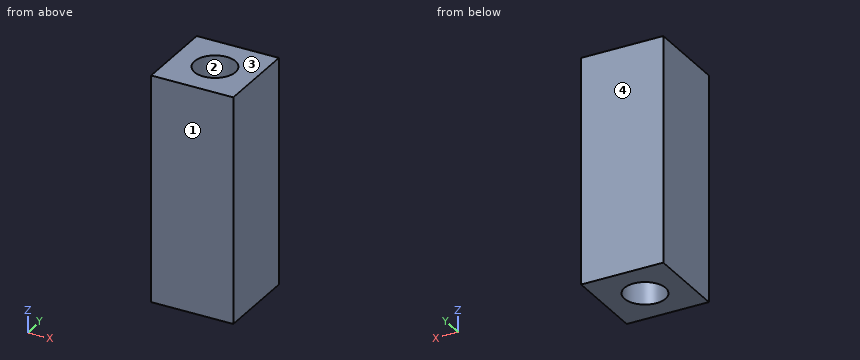
```python
from build123d import *

# Parameters (mm, degrees)
F1_DEPTH = 279.4


with BuildPart() as f1:
    # F0 (on Top) → F1 (new body)
    with BuildSketch(Plane.XY):
        with BuildLine():
            ThreePointArc((-25.4, 0), (0, 25.4), (25.4, 0))
            Line((25.4, 0), (50.8, 0))
            Line((50.8, 0), (50.8, 50.8))
            Line((50.8, 50.8), (-50.8, 50.8))
            Line((-50.8, 50.8), (-50.8, 0))
            Line((-50.8, 0), (-25.4, 0))
        make_face()
        with BuildLine():
            Line((50.8, 0), (25.4, 0))
            ThreePointArc((25.4, 0), (0, -25.4), (-25.4, 0))
            Line((-25.4, 0), (-50.8, 0))
            Line((-50.8, 0), (-50.8, -50.8))
            Line((-50.8, -50.8), (50.8, -50.8))
            Line((50.8, -50.8), (50.8, 0))
        make_face()
    extrude(amount=F1_DEPTH)


solid = f1.part
```
Geometry check sheet. Reference: the model listing, model coordinates, mm. Face numbers are marked on the shaded views. Coordinates: 2 decimals unless noted, no trailing zeros. Order: outer loops, then holes, each group sorted by start corner. A loop starts at its lowest first (then second) coordinate and runs counter-clockwise, first axis right, second up. Notation, with made-up numbers: M 69,74.5 L 73,74.5 A22 ccw 73,81.5 Z; hole C 44.5,4.5 d4. An arc over 180 degrees is marked long. Answer as a JSON object with one key per item and string values.
Q1. Scan lines: line 1 (Y direction, x = 0, z = 170.5); line 2 (Y direction, x = -12, z = 33.5); line 3 (X direction, y = -11.5, z = 39.5). Record each from-to range of solid material in increasing order.
Results are:
{"line 1": "y = -50.8 to -25.4, 25.4 to 50.8", "line 2": "y = -50.8 to -22.39, 22.39 to 50.8", "line 3": "x = -50.8 to -22.65, 22.65 to 50.8"}
Q2. Cross-section at C-C on z = 173.5. Record the cut outline in (x, y).
Results are:
{"outline": "M -50.8,-50.8 L 50.8,-50.8 L 50.8,50.8 L -50.8,50.8 Z; hole C 0,0 d50.8"}
Q3. Depth check by flat-ended pin: pin 1 Ø6 at (x, y) = (-18, 26.5) entering from -Z. Enter the tip coordinate at first touch or a pass-through.
Results are:
{"pin 1": "stops at z = 0"}
Q4. Release check for a two-part mould opening along Y. For the marked faces 1, 2, 3 and 4 record: released by +Y, released by -Y, zero draft, split by the parting line, or undercut.
Results are:
{"face 1": "released by -Y", "face 2": "undercut", "face 3": "zero draft", "face 4": "released by +Y"}
Q5. Cross-section at A-A on y = 0. Record the cut outline in (x, z).
Results are:
{"outline": "M -50.8,0 L -25.4,0 L -25.4,279.4 L -50.8,279.4 Z; M 25.4,0 L 50.8,0 L 50.8,279.4 L 25.4,279.4 Z"}
